```python
from build123d import *

# Parameters (mm, degrees)
ESBO_O1_R                = 82.5
ESBO_O1_R_2              = 14
RESSALTO_EXTRUS_O1_DEPTH = 3
ESBO_O2_R                = 5.925
RESSALTO_EXTRUS_O2_DEPTH = 8
ESBO_O3_R                = 14
RESSALTO_EXTRUS_O3_DEPTH = 3
ESBO_O4_R                = 10
RESSALTO_EXTRUS_O4_DEPTH = 11
ESBO_O5_R                = 3.05
CORTE_EXTRUS_O1_DEPTH    = 1
ESBO_O6_R                = 76.5
RESSALTO_EXTRUS_O5_DEPTH = 7
ESBO_O13_R               = 2
CORTE_EXTRUS_O2_DEPTH    = 11
ESBO_O14_R               = 7.5
CORTE_EXTRUS_O3_DEPTH    = 5


with BuildPart() as part:
    # Esboço1 → Ressalto-extrusão1 (new body)
    with BuildSketch(Plane.XY):
        Circle(ESBO_O1_R)
        Circle(ESBO_O1_R_2, mode=Mode.SUBTRACT)
    extrude(amount=RESSALTO_EXTRUS_O1_DEPTH)

    # Esboço2 → Ressalto-extrusão2 (add)
    with BuildSketch(Plane(origin=(0, 0, 0), x_dir=(-1, 0, 0), z_dir=(0, 0, -1))):
        with Locations((-55.155254038, 14.383947721)):
            Circle(ESBO_O2_R)
        with Locations((40.034491152, 40.573877288)):
            Circle(ESBO_O2_R)
        with Locations((15.120762886, -54.957825009)):
            Circle(ESBO_O2_R)
    extrude(amount=RESSALTO_EXTRUS_O2_DEPTH)

    # Esboço3 → Ressalto-extrusão3 (add)
    with BuildSketch(Plane.XY.offset(3)):
        Circle(ESBO_O3_R)
    extrude(amount=-RESSALTO_EXTRUS_O3_DEPTH)

    # Esboço4 → Ressalto-extrusão4 (add)
    with BuildSketch(Plane.XY.offset(3)):
        Circle(ESBO_O4_R)
    extrude(amount=-RESSALTO_EXTRUS_O4_DEPTH)

    # Esboço5 → Corte-extrusão1 (cut)
    with BuildSketch(Plane(origin=(0, 0, -8), x_dir=(-1, 0, 0), z_dir=(0, 0, -1))):
        Circle(ESBO_O5_R)
    extrude(amount=-CORTE_EXTRUS_O1_DEPTH, mode=Mode.SUBTRACT)

    # Esboço6 → Ressalto-extrusão5 (add)
    with BuildSketch(Plane.XY.offset(3)):
        Circle(ESBO_O6_R)
    extrude(amount=RESSALTO_EXTRUS_O5_DEPTH)

    # Esboço13 → Corte-extrusão2 (cut, through all)
    with BuildSketch(Plane(origin=(0, 0, 0), x_dir=(-1, 0, 0), z_dir=(0, 0, -1))):
        with Locations((-1.573494017, -55.549458165)):
            Circle(ESBO_O13_R)
        with Locations((26.098018566, -30.463408429)):
            Circle(ESBO_O13_R)
        with Locations((53.76953115, -5.377358693)):
            Circle(ESBO_O13_R)
        with Locations((-51.407244113, -0.579653936)):
            Circle(ESBO_O13_R)
        with Locations((-23.73573153, 24.5063958)):
            Circle(ESBO_O13_R)
        with Locations((3.935781053, 49.592445536)):
            Circle(ESBO_O13_R)
    extrude(amount=-CORTE_EXTRUS_O2_DEPTH, mode=Mode.SUBTRACT)

    # Esboço14 → Corte-extrusão3 (cut)
    with BuildSketch(Plane(origin=(0, 0, 0), x_dir=(-1, 0, 0), z_dir=(0, 0, -1))):
        with Locations((53.76953115, -5.377358693)):
            Circle(ESBO_O14_R)
        with Locations((26.098018566, -30.463408429)):
            Circle(ESBO_O14_R)
        with Locations((-1.573494017, -55.549458165)):
            Circle(ESBO_O14_R)
        with Locations((3.935781053, 49.592445536)):
            Circle(ESBO_O14_R)
        with Locations((-23.73573153, 24.5063958)):
            Circle(ESBO_O14_R)
        with Locations((-51.407244113, -0.579653936)):
            Circle(ESBO_O14_R)
    extrude(amount=-CORTE_EXTRUS_O3_DEPTH, mode=Mode.SUBTRACT)


solid = part.part
```
Here's how the part is built. I have some questions about the finished solid (model axes, mm). A direction names the side the tool comes from. Coordinates: 2 decimals unless noted, no trailing zeros. Order: outer loops, then holes, each group sorted by start corner. A loop starts at its lowest first (then second) coordinate and runs counter-clockwise, first axis right, second up. Notation, with made-up numbers: (31.5, -28) - (63.5, -28) arc R16 cw to (63.5, -23) - close; hole circle Ø7 at (44.25, 8). An arc over 180 degrees is marked (long way). One line per question, with ' | ' between items. Start each with the question number.
1. If we section it at C-C (z = -3): Give the number of separate pieces and of enclosed holes in the cut face, and give its area (3 significant figures).
2. If we mould it in two halves opening along Y, with no side actions, what happens to faces 1 (the flat face through (55, 14, -8)), 2 (the cylindrical face through (49.682, 12.115, -3.944)), 3 (the cylindrical face through (25.362, 17.185, 2.465))? For each: released by +Y, released by -Y, zero draft, split by the parting line, or undercut.
3. I'm going to push flat-ended pins straight in: pin 1 Ø19.5 at (x, y) = (-3.94, 49.59) entering from +Z; pin 2 Ø4 at (y, z) = (28, -0.5) entering from +X; pin 3 Ø1 at (x, z) = (64.5, 1.5) entering from -Y; pin 4 Ø4 at (x, z) = (-21, -1.5) entering from +Y. Where does each tip first touch, or does it pass through?
4. If we section it at B-B (y = -70): Write out the boundary of the cut face in (x, z), and give its area (3 significant figures).
5. Which directions (+Z, -Z, +X, -X, +Y, -Y) give clear straight access to the entire face, cutting with the end or side of a thin tool? Please do faces 4 (the cylindrical face through (-2.31, 42.27, 2.46)), 5 (the cylindrical face through (-60.708, -46.549, 6.451)), 6 (the cylindrical face through (53.405, -0.492, 7.465)).
6. If we section it at D-D (x = -39): Write out the boundary of the cut face in (y, z), and give its area (3 significant figures).
7. Please list where these lines run through material, in increasing order: line 1 along X through (y, z) = (-3, 2.25); line 2 along Z through (x, y) = (2, 59); line 3 along Z through (x, y) = (-32.5, -73.5). Write a range as [from, to].
8. If we section it at A-A (x = 13.5): Write out the boundary of the cut face in (y, z).
Model answer:
1) separate pieces: 4 | enclosed holes: 0 | area: 645 mm²
2) face 1: zero draft | face 2: split by the parting line | face 3: undercut
3) pin 1: stops at z = 10 | pin 2: stops at x = 78.27 | pin 3: stops at y = -52.06 | pin 4: stops at y = 80.12
4) outline: (-43.66, 0) - (43.66, 0) - (43.66, 3) - (30.86, 3) - (30.86, 10) - (-30.86, 10) - (-30.86, 3) - (-43.66, 3) - close | area: 694 mm²
5) face 4: -Z | face 5: +Z | face 6: +Z, -Z
6) outline: (-72.7, 0) - (34.74, 0) - (34.74, -8) - (46.41, -8) - (46.41, 0) - (72.7, 0) - (72.7, 3) - (65.81, 3) - (65.81, 10) - (-65.81, 10) - (-65.81, 3) - (-72.7, 3) - close | area: 1,450 mm²
7) line 1: x = [-82.45, -60.88], [-46.66, 44.31], [58.51, 82.45] | line 2: z = [0, 10] | line 3: z = [0, 3]
8) outline: (-81.39, 0) - (81.39, 0) - (81.39, 3) - (75.3, 3) - (75.3, 10) - (-75.3, 10) - (-75.3, 3) - (-81.39, 3) - close
